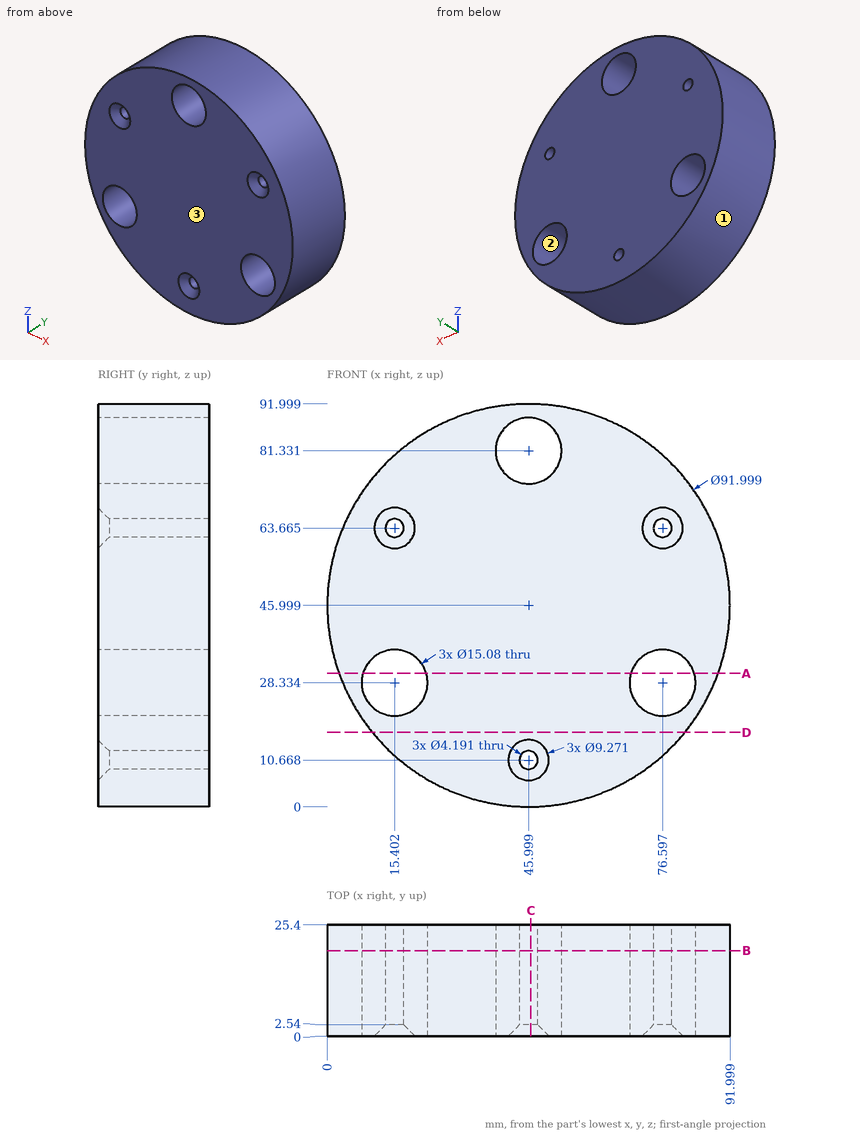
Design review of the part shown in the three views and the two pictorial views. Dimensions are in mm from the part's minimum x, y and z. Round coordinates to 2 decimals unless told otherwise and drop trailing zeros. Write each loop counter-clockwise with the first axis right and the second up, starting at its lowest first coordinate (ties: lowest second). Pieces come first, ordered by that corner, then holes.
1) Take a section at A-A on z = 30.5. Give the boundary of the cut face in (x, y) (1 decimal), then the cut area to 3 significant figures.
Answer below:
outline: (2.7, 0) - (8.2, 0) - (8.2, 25.4) - (2.7, 25.4) - close; (22.6, 0) - (69.4, 0) - (69.4, 25.4) - (22.6, 25.4) - close; (83.8, 0) - (89.3, 0) - (89.3, 25.4) - (83.8, 25.4) - close
area: 1,470 mm2
2) For line 1 along Z through (x, y) = (47, 17.25) (1 decimal); line 2 along X through (y, z) = (18.75, 25.5) (1 decimal); line 3 along X through (y, z) = (20, 32.5) (1 decimal), list the stretches that pass through material, from the lowest coordinate up.
Answer below:
line 1: z = 0 to 8.8, 12.5 to 73.9, 88.8 to 92
line 2: x = 4.8 to 8.4, 22.4 to 69.6, 83.6 to 87.2
line 3: x = 2 to 9.1, 21.7 to 70.3, 82.9 to 90
3) Mouldability with a two-part tool opening along X and no side actions: class the marked faces 1, 2 and 3 as +X half, -X half, draft (parallel to the pull), parting line (faces both ways), or undercut.
Answer below:
face 1: parting line
face 2: undercut
face 3: draft
4) Take a section at B-B on y = 19.5. Give the boundary of the cut face in (x, z) (1 decimal), then the cut area to 3 significant figures.
Answer below:
outline: circle Ø92 at (46, 46); hole circle Ø15.1 at (15.4, 28.3); hole circle Ø4.2 at (15.4, 63.7); hole circle Ø15.1 at (46, 81.3); hole circle Ø4.2 at (46, 10.7); hole circle Ø15.1 at (76.6, 28.3); hole circle Ø4.2 at (76.6, 63.7)
area: 6,070 mm2
5) Take a section at D-D on z = 17. Give the boundary of the cut face in (x, y).
Answer below:
outline: (10.29, 0) - (81.71, 0) - (81.71, 25.4) - (10.29, 25.4) - close
6) Insertion check: pin 1 Ø4 at (y, z) = (19.5, 25.5) entering from +X (1 decimal); pin 2 Ø13.5 at (x, z) = (76.6, 28.33) entering from -Y; pin 3 Ø5 at (y, z) = (19, 33.5) entering from +X; pin 4 Ø2 at (y, z) = (14.5, 27.5) entering from +X. Each pin has a flat end and moves straight along its axis. Give the tip position at first contact, or say it passes through.
Answer below:
pin 1: stops at x = 88.1
pin 2: passes through
pin 3: stops at x = 90.9
pin 4: stops at x = 88.54
7) Take a section at C-C on x = 46.5. State how many separate pieces and enclosed holes the cut face has, then the cut area to 3 significant figures.
Answer below:
separate pieces: 3
enclosed holes: 0
area: 1,840 mm2
